For this review, take the finished solid that the model builds, in its own axes (mm). Face numbers are marked on the shaded views. A direction names the side the tool comes from. Coordinates: 2 decimals unless noted, no trailing zeros. Order: outer loops, then holes, each group sorted by start corner. A loop starts at its lowest first (then second) coordinate and runs counter-clockwise, first axis right, second up. Notation, with made-up numbers: M 47.5,26 L 66.5,26 A26 ccw 66.5,44 Z; hole C 25.5,-23.75 d8. An arc over 180 degrees is marked long. Use CSV: the item, a comma, the result in double quotes.
```python
from build123d import *

# Parameters (mm, degrees)
CUT_EXTRUDE1_DEPTH = 1.3
FILLET1_R          = 0.1
CUT_EXTRUDE2_START = -0.5
SKETCH3_R          = 1.8
SKETCH3_R_2        = 1.7
CUT_EXTRUDE2_DEPTH = 0.5


with BuildPart() as part:
    # Sketch1 → Revolve1 (revolve)
    with BuildSketch(Plane(origin=(0, 0, 0), x_dir=(0, 0, -1), z_dir=(1, 0, 0))):
        Polygon((0, 0), (0, -23.8), (1, -23.8), (1, -1.8), (1.8, -1.8), (1.8, 0), align=None)
    revolve(axis=Axis((0, 0, 0), (0, 1, 0)))

    # Sketch2 → Cut-Extrude1 (cut)
    with BuildSketch(Plane(origin=(0, 0, 0), x_dir=(1, 0, 0), z_dir=(0, 1, 0))):
        Polygon((0, 0.866025404), (-0.75, 0.433012702), (-0.75, -0.433012702), (0, -0.866025404), (0.75, -0.433012702), (0.75, 0.433012702), align=None)
    extrude(amount=-CUT_EXTRUDE1_DEPTH, mode=Mode.SUBTRACT)

    # Fillet1
    fillet1_edges = [part.edges().sort_by_distance(p)[0] for p in [
        (0, 0, 1.8),
    ]]
    fillet(fillet1_edges, radius=FILLET1_R)

    # Sketch3 → Cut-Extrude2 (cut)
    with BuildSketch(Plane.XZ.offset(1.8).offset(CUT_EXTRUDE2_START)):
        with Locations(Location((0, 0, 0), (0, 0, 270))):
            Circle(SKETCH3_R)
        with Locations(Location((0, 0, 0), (0, 0, 270))):
            Circle(SKETCH3_R_2, mode=Mode.SUBTRACT)
    extrude(amount=CUT_EXTRUDE2_DEPTH, mode=Mode.SUBTRACT)


solid = part.part
```
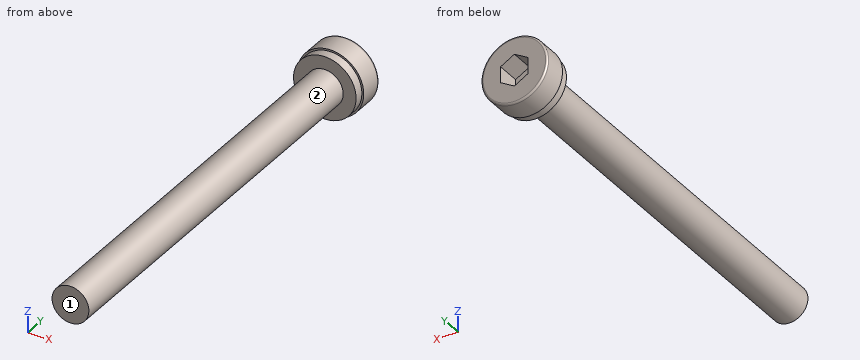
Item 1: Add section A-A on z = 0. State the section outline as (x, y) points.
Solutions:
outline,"M -1.8,-1.3 L -1.7,-1.3 L -1.7,-1.8 L -1,-1.8 L -1,-23.8 L 1,-23.8 L 1,-1.8 L 1.7,-1.8 L 1.7,-1.3 L 1.8,-1.3 L 1.8,-0.1 A0.1 ccw 1.7,0 L 0.75,0 L 0.75,-1.3 L -0.75,-1.3 L -0.75,0 L -1.7,0 A0.1 ccw -1.8,-0.1 Z"
Item 2: Add section B-B on y = -2.25. State the section outline as (x, z) points, and give its area (3 significant figures).
Solutions:
outline,"C 0,0 d2"
area,"3.14 mm^2"
Item 3: For the marked faces 1 and 2, list the 3-axis set-ups (+Z, -Z, +X, -X, +Y, -Y) from which the entire face can be reached by the end or side of a thin tool; tool diameter is ignored.
Solutions:
face 1,"+Z, -Z, +X, -X, -Y"
face 2,"-Y"
Item 4: To check wall thickness, follow line 1 along Y through (x, z) = (0.4, 1.15); line 2 along Y through (x, z) = (0.6, -0.4); line 3 along Z through (x, y) = (-0.5, -14.5). State the ranges of each line that lie inside material, in increasing order. Write a range as [from, to].
Solutions:
line 1,"[-1.8, 0]"
line 2,"[-23.8, -1.3]"
line 3,"[-0.87, 0.87]"
Item 5: Clearance check with flat-ended pins moving along their axes: pin 1 Ø0.5 at (x, z) = (0, 0.5) entering from +Y; pin 2 Ø1.5 at (x, z) = (-0.5, 1) entering from +Y; pin 3 Ø1 at (y, z) = (-17, 1) entering from +X; pin 4 Ø1 at (y, z) = (-11.5, 0.5) entering from -X. State where each tip first meets the part, or that it passes through.
Solutions:
pin 1,"y = -1.3"
pin 2,"y = 0"
pin 3,"x = 0.87"
pin 4,"x = -1"
